```python
from build123d import *

# Parameters (mm, degrees)
SKETCH1_W           = 134.1999983
SKETCH1_H           = 59.69999998
BOSS_EXTRUDE1_DEPTH = 1.12
BOSS_EXTRUDE2_DEPTH = 7


with BuildPart() as part:
    # Sketch1 → Boss-Extrude1 (new body)
    with BuildSketch(Plane.XY):
        with Locations((145.59999963, 116.24999991)):
            Rectangle(SKETCH1_W, SKETCH1_H)
    extrude(amount=BOSS_EXTRUDE1_DEPTH)

    # Sketch2 → Boss-Extrude2 (add)
    with BuildSketch(Plane.XY.offset(1.12)):
        Polygon((161.3255092, 89.07300956), (196.57449128, 89.02550902), (196.37449168, 144.37449154), (161.3255092, 144.37449154), align=None)
    extrude(amount=BOSS_EXTRUDE2_DEPTH)


solid = part.part
```
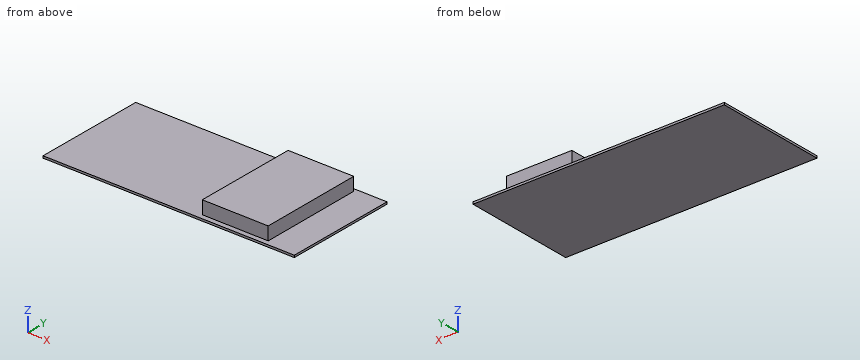
Can you work these out from the model? Positions are in its coordinate system, mm. Give positions to 0.01 mm unless a question says otherwise; leave off trailing zeros. Order: outer loops, then holes, each group sorted by start corner. A loop starts at its lowest first (then second) coordinate and runs counter-clockwise, first axis right, second up. Notation, with made-up numbers: M -25.75,-29.75 L 0.25,-29.75 A18 cw 0.25,-15.75 Z; hole C -26,-26 d5. An arc over 180 degrees is marked long. Write item = value, one per line. Start each with the question number.
Q1. Will these pins go through, and if not, where does the flat tip stop? pin 1 Ø1.5 at (x, z) = (195, 4) entering from +Y; pin 2 Ø3 at (x, y) = (105, 139) entering from +Z; pin 3 Ø2 at (y, z) = (105.5, 7) entering from -X.
Q2. Suppose I cut it at C-C (z = 3.75). Write out the boundary of the cut face in (x, y).
Q3. Suppose I cut it at A-A (y = 117). Write out the boundary of the cut face in (x, z), plus the area to 3 significant figures.
Q4. Suppose I cut it at D-D (x = 203). Write out the boundary of the cut face in (y, z).
Q5. I need wall thicknesses on probe 1 along X at (y, z) = (95, 5.75); probe 2 along Z at (x, y) = (159.5, 98); probe 3 along Y at (x, z) = (177, 7). Which ranges of each line are inside material? Lowest first, please. Write a range as [from, to].
Q6. Suppose I cut it at B-B (x = 171). Write out the boundary of the cut face in (y, z).
Check result:
q1.pin_1 = 144.37
q1.pin_2 = 1.12
q1.pin_3 = 161.33
q2.outline = M 161.33,89.07 L 196.57,89.03 L 196.37,144.37 L 161.33,144.37 Z
q3.outline = M 78.5,0 L 212.7,0 L 212.7,1.12 L 196.47,1.12 L 196.47,8.12 L 161.33,8.12 L 161.33,1.12 L 78.5,1.12 Z
q3.area = 396 mm2
q4.outline = M 86.4,0 L 146.1,0 L 146.1,1.12 L 86.4,1.12 Z
q5.probe_1 = [161.33, 196.55]
q5.probe_2 = [0, 1.12]
q5.probe_3 = [89.05, 144.37]
q6.outline = M 86.4,0 L 146.1,0 L 146.1,1.12 L 144.37,1.12 L 144.37,8.12 L 89.06,8.12 L 89.06,1.12 L 86.4,1.12 Z
